```python
from build123d import *

# Parameters (mm, degrees)
SKETCH_1_W          = 4
SKETCH_1_H          = 4
EXTRUDE_1_DEPTH     = 30
SKETCH_3_W          = 8
SKETCH_3_H          = 2
CUT_EXTRUDE_1_DEPTH = 2
SKETCH_5_W          = 2
SKETCH_5_H          = 2
CUT_EXTRUDE_2_DEPTH = 2
SKETCH_6_W          = 2
SKETCH_6_H          = 2
CUT_EXTRUDE_3_DEPTH = 2
SKETCH_8_W          = 2
SKETCH_8_H          = 4
CUT_EXTRUDE_4_DEPTH = 2


with BuildPart() as part:
    # 草圖1 → 填料-伸長1 (new body)
    with BuildSketch(Plane.XY):
        Rectangle(SKETCH_1_W, SKETCH_1_H)
    extrude(amount=EXTRUDE_1_DEPTH)

    # 草圖3 → 除料-伸長1 (cut)
    with BuildSketch(Plane.ZY.offset(2)):
        with Locations((15, -1)):
            Rectangle(SKETCH_3_W, SKETCH_3_H)
    extrude(amount=-CUT_EXTRUDE_1_DEPTH, mode=Mode.SUBTRACT)

    # 草圖5 → 除料-伸長2 (cut)
    with BuildSketch(Plane.ZY):
        with Locations((18, -1)):
            Rectangle(SKETCH_5_W, SKETCH_5_H)
    extrude(amount=-CUT_EXTRUDE_2_DEPTH, mode=Mode.SUBTRACT)

    # 草圖6 → 除料-伸長3 (cut)
    with BuildSketch(Plane.ZY):
        with Locations((12, -1)):
            Rectangle(SKETCH_6_W, SKETCH_6_H)
    extrude(amount=-CUT_EXTRUDE_3_DEPTH, mode=Mode.SUBTRACT)

    # 草圖8 → 除料-伸長4 (cut)
    with BuildSketch(Plane.XZ):
        with Locations((-1, 15)):
            Rectangle(SKETCH_8_W, SKETCH_8_H)
    extrude(amount=-CUT_EXTRUDE_4_DEPTH, mode=Mode.SUBTRACT)


solid = part.part
```
Check sheet for the modelled part. Datum: model origin and axes. Units: mm. A direction names the side the tool comes from. Round coordinates to 2 decimals unless told otherwise and drop trailing zeros. Loops run counter-clockwise (first coordinate to the right, second up) from the corner with the lowest first, then second, coordinate; pieces in that order, holes last. Notation, with made-up numbers: (-37.5, -18.5) -> (-10.5, -18.5) arc R8 cw to (-10.5, -8.5) -> close; hole circle Ø7 at (76.25, 27). An arc over 180 degrees is marked (long way). Answer in a Markdown table with one row per item.
Q1. Thickness scan on L1, parallel to Z at x = 1.3, y = -0.2; L2, parallel to Z at x = -1, y = -1.3; L3, parallel to X at y = -0.55, z = 16. Record the ranges inside material, lowest first.
Data:
| item | result |
|---|---|
| L1 | z = 0 to 11, 13 to 17, 19 to 30 |
| L2 | z = 0 to 11, 19 to 30 |
| L3 | x = 0 to 2 |
Q2. Sectioned sample at A-A on x = -1.6. Enter the section's corners in (y, z).
Data:
| item | result |
|---|---|
| outline | (-2, 0) -> (2, 0) -> (2, 13) -> (0, 13) -> (0, 11) -> (-2, 11) -> close; (-2, 19) -> (0, 19) -> (0, 17) -> (2, 17) -> (2, 30) -> (-2, 30) -> close |
Q3. Sectioned sample at C-C on y = 1.6. Enter the section's corners in (x, z).
Data:
| item | result |
|---|---|
| outline | (-2, 0) -> (2, 0) -> (2, 30) -> (-2, 30) -> (-2, 17) -> (0, 17) -> (0, 13) -> (-2, 13) -> close |
Q4. Release check for a two-part mould opening along Z. For faces 4 (the face through (1, -1, 13)), 5 (the face through (0, 0, 12)), 6 (the face through (0, 0, 30)), 7 (the face through (-2, 0, 6)) record: released by +Z, released by -Z, zero draft, split by the parting line, or undercut.
Data:
| item | result |
|---|---|
| face 4 | undercut |
| face 5 | undercut |
| face 6 | released by +Z |
| face 7 | zero draft |
Q5. Go/stop test with flat-tipped pins: P1, Ø1.6, axis at x = 1, z = 18, coming from the -Y side; P2, Ø2, axis at y = -0.5, z = 14.5, coming from the -X side. Record where each tip stops, or that it passes through.
Data:
| item | result |
|---|---|
| P1 | stops at y = 0 |
| P2 | stops at x = 0 |
Q6. Sectioned sample at D-D on x = 1.45. Enter the section's corners in (y, z).
Data:
| item | result |
|---|---|
| outline | (-2, 0) -> (2, 0) -> (2, 30) -> (-2, 30) -> (-2, 19) -> (0, 19) -> (0, 17) -> (-2, 17) -> (-2, 13) -> (0, 13) -> (0, 11) -> (-2, 11) -> close |
Q7. Sectioned sample at B-B on y = -0.65. Enter the section's corners in (x, z).
Data:
| item | result |
|---|---|
| outline | (-2, 0) -> (2, 0) -> (2, 11) -> (-2, 11) -> close; (-2, 19) -> (2, 19) -> (2, 30) -> (-2, 30) -> close; (0, 13) -> (2, 13) -> (2, 17) -> (0, 17) -> close |
Q8. Set-up check for faces 1 (the face through (0, 0, 18)), 2 (the face through (1, -2, 15)), 3 (the face through (0, 0, 15)): record each of +Z, -Z, +X, -X, +Y, -Y from which the full face is reachable in a straight line by a thin tool's end or side.
Data:
| item | result |
|---|---|
| face 1 | +X, -X, -Y |
| face 2 | +Z, -Z, +X, -X, -Y |
| face 3 | -X, +Y, -Y |
